Input: dimensioned drawing with shaded views. Units: mm. Origin: part minimum x, y, z. A direction names the side the tool comes from. Round coordinates to 2 decimals unless told otherwise and drop trailing zeros. Order: outer loops, then holes, each group sorted by start corner. A loop starts at its lowest first (then second) coordinate and runs counter-clockwise, first axis right, second up. Notation, with made-up numbers: (65.5, -27) - (75.5, -27) arc R23 ccw to (75.5, -11) - close; hole circle Ø7 at (8, -26). An arc over 180 degrees is marked (long way). Return JSON: item names as keys, results as strings. Group by question number.
1) Section A-A, the plane y = 4.75. Return loops of the section in (x, z).
2) Section D-D, the plane z = 2.5. Return loops of the section in (x, y).
3) Section B-B, the plane z = 29.5. Return loops of the section in (x, y).
4) Section C-C, the plane x = 84.5. Return loops of the section in (y, z).
5) Ray query, line 1 (Y direction, x = 18, z = 33.5); line 2 (Z direction, x = 14.5, y = 7); line 3 (X direction, y = 6, z = 23). Return the intervals inside material, ascending. Write a range as from..to.
6) Contact query for flat-ended pins moving along their axis: P1, Ø4, axis at y = 6.5, z = 4.5, coming from the -X side; P2, Ø1.5, axis at x = 53.5, y = 4.5, coming from the +Z side; P3, Ø1, axis at x = 10.5, y = 2, coming from the -Z side; P4, Ø2.5, axis at x = 45.5, y = 5.5, coming from the -Z side. Output: stop coordinate, or through.
7) Access query for the marked faces 1, 2, 3, 4 and 5. Directions: +Z, -Z, +X, -X, +Y, -Y. A direction counts if a zero-diameter tool reaches every point of the face in a straight line with its end or side. Return the directions, or none.
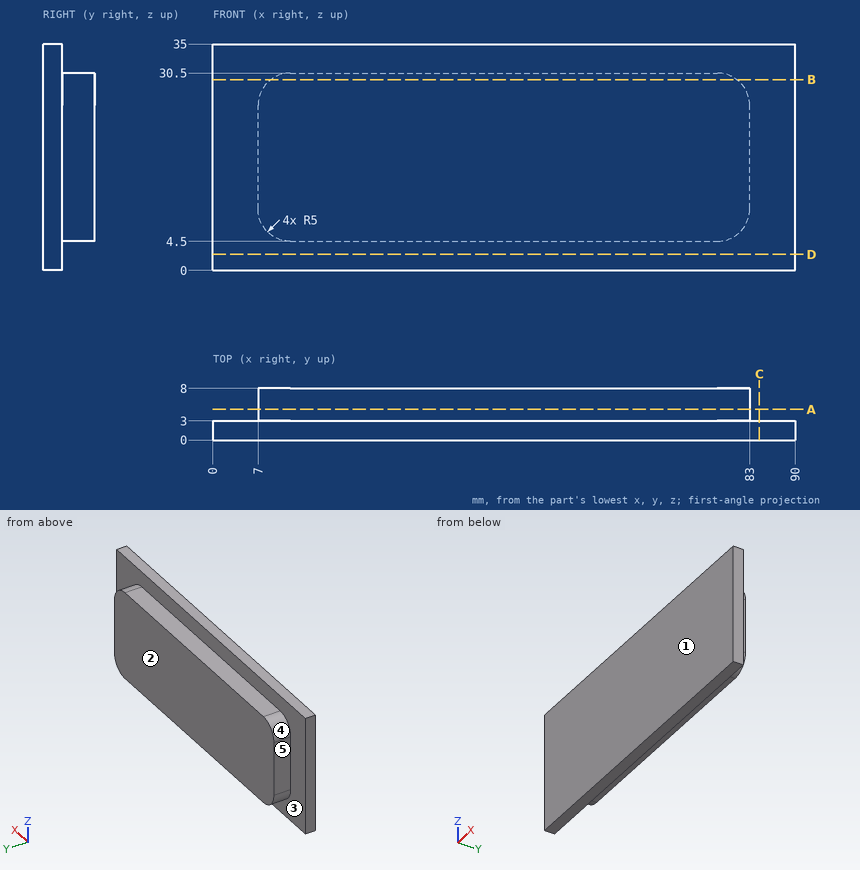
Geometry check:
{
 "1": {"outline": "(7, 9.5) arc R5 ccw to (12, 4.5) - (78, 4.5) arc R5 ccw to (83, 9.5) - (83, 25.5) arc R5 ccw to (78, 30.5) - (12, 30.5) arc R5 ccw to (7, 25.5) - close"},
 "2": {"outline": "(0, 0) - (90, 0) - (90, 3) - (0, 3) - close"},
 "3": {"outline": "(0, 0) - (90, 0) - (90, 3) - (81, 3) - (81, 8) - (9, 8) - (9, 3) - (0, 3) - close"},
 "4": {"outline": "(0, 0) - (3, 0) - (3, 35) - (0, 35) - close"},
 "5": {"line 1": "0..3", "line 2": "4.5..30.5", "line 3": "7..83"},
 "6": {"P1": "x = 8", "P2": "z = 30.5", "P3": "z = 0", "P4": "z = 4.5"},
 "7": {"face 1": "+Z, -Z, +X, -X, -Y", "face 2": "+Z, -Z, +X, -X, +Y", "face 3": "+Y", "face 4": "+Z, -X, +Y", "face 5": "+Z, -Z, -X, +Y"}
}
